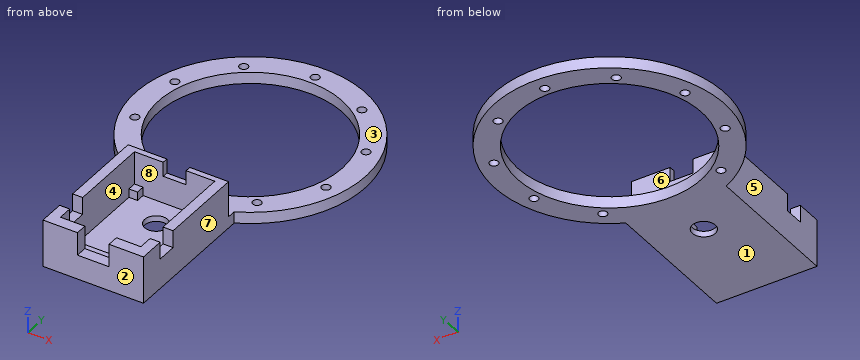
```python
from build123d import *

# Parameters (mm, degrees)
SKETCH1_R             = 1.5
SKETCH1_R_2           = 32
BOSS_EXTRUDE1_DEPTH   = 4
SKETCH1_3_R           = 4
BOSS_EXTRUDE2_DEPTH   = 2
SKETCH1_11_W          = 28
SKETCH1_11_H          = 6
BOSS_EXTRUDE4_DEPTH   = 5
SKETCH1_11_W_2        = 3
SKETCH1_11_H_2        = 3
BOSS_EXTRUDE4_2_DEPTH = 5
BOSS_EXTRUDE4_3_DEPTH = 5
SKETCH1_21_W          = 35
SKETCH1_21_H          = 46
BOSS_EXTRUDE7_DEPTH   = 16.5
SKETCH3_W             = 6
SKETCH3_H             = 7
CUT_EXTRUDE1_DEPTH    = 35.5
SKETCH4_W             = 11
SKETCH4_H             = 8
CUT_EXTRUDE2_DEPTH    = 4
SKETCH5_W             = 8
SKETCH5_H             = 5
CUT_EXTRUDE3_DEPTH    = 52


with BuildPart() as part:
    # Sketch1 → Boss-Extrude1 (new body)
    with BuildSketch(Plane.XY):
        with BuildLine():
            Line((-17.5, -38.96998799), (17.5, -38.96998799))
            Line((17.5, -38.96998799), (17.5, -35.968736425))
            ThreePointArc((17.5, -35.968736425), (0, 40), (-17.5, -35.968736425))
            Line((-17.5, -35.968736425), (-17.5, -38.96998799))
        make_face()
        with Locations((-20.57248383, -28.315594803)):
            Circle(SKETCH1_R, mode=Mode.SUBTRACT)
        with Locations((20.57248383, -28.315594803)):
            Circle(SKETCH1_R, mode=Mode.SUBTRACT)
        with Locations((-33.28697807, -10.815594803)):
            Circle(SKETCH1_R, mode=Mode.SUBTRACT)
        Circle(SKETCH1_R_2, mode=Mode.SUBTRACT)
        with Locations((-33.28697807, 10.815594803)):
            Circle(SKETCH1_R, mode=Mode.SUBTRACT)
        with Locations((-20.57248383, 28.315594803)):
            Circle(SKETCH1_R, mode=Mode.SUBTRACT)
        with Locations((0, 35)):
            Circle(SKETCH1_R, mode=Mode.SUBTRACT)
        with Locations((33.28697807, -10.815594803)):
            Circle(SKETCH1_R, mode=Mode.SUBTRACT)
        with Locations((33.28697807, 10.815594803)):
            Circle(SKETCH1_R, mode=Mode.SUBTRACT)
        with Locations((20.57248383, 28.315594803)):
            Circle(SKETCH1_R, mode=Mode.SUBTRACT)
    extrude(amount=BOSS_EXTRUDE1_DEPTH)



with BuildPart() as body_2:
    # Sketch1<3> → Boss-Extrude2 (new body)
    with BuildSketch(Plane.XY):
        Polygon((11, -40.96998799), (-11, -40.96998799), (-11, -43.96998799), (-14, -43.96998799), (-14, -74.96998799), (14, -74.96998799), (14, -43.96998799), (11, -43.96998799), align=None)
        with Locations((0, -50.96998799)):
            Circle(SKETCH1_3_R, mode=Mode.SUBTRACT)
    extrude(amount=BOSS_EXTRUDE2_DEPTH)


with BuildPart() as body_3:
    # Sketch1<11> → Boss-Extrude4 (new body)
    with BuildSketch(Plane.XY):
        with Locations((0, -77.96998799)):
            Rectangle(SKETCH1_11_W, SKETCH1_11_H)
    extrude(amount=BOSS_EXTRUDE4_DEPTH)


with BuildPart() as body_4:
    # Sketch1<11> → Boss-Extrude4 2 (new body)
    with BuildSketch(Plane.XY):
        with Locations((-12.5, -42.46998799)):
            Rectangle(SKETCH1_11_W_2, SKETCH1_11_H_2)
    extrude(amount=BOSS_EXTRUDE4_2_DEPTH)


with BuildPart() as body_5:
    # Sketch1<11> → Boss-Extrude4 3 (new body)
    with BuildSketch(Plane.XY):
        with Locations((12.5, -42.46998799)):
            Rectangle(SKETCH1_11_W_2, SKETCH1_11_H_2)
    extrude(amount=BOSS_EXTRUDE4_3_DEPTH)


with BuildPart() as part_1:
    add(part.part)

    add(body_2.part)  # Boss-Extrude7 merges body 2

    add(body_3.part)  # Boss-Extrude7 merges body 3

    add(body_4.part)  # Boss-Extrude7 merges body 4

    add(body_5.part)  # Boss-Extrude7 merges body 5
    # Sketch1<21> → Boss-Extrude7 (add)
    with BuildSketch(Plane.XY):
        with Locations((0, -61.96998799)):
            Rectangle(SKETCH1_21_W, SKETCH1_21_H)
        Polygon((-14, -43.96998799), (-14, -40.96998799), (-11, -40.96998799), (11, -40.96998799), (14, -40.96998799), (14, -43.96998799), (14, -74.96998799), (14, -80.96998799), (-14, -80.96998799), (-14, -74.96998799), align=None, mode=Mode.SUBTRACT)
    extrude(amount=BOSS_EXTRUDE7_DEPTH)

    # Sketch3 → Cut-Extrude1 (cut)
    with BuildSketch(Plane(origin=(17.5, 0, 0), x_dir=(0, 0, -1), z_dir=(1, 0, 0))):
        with Locations((-13.5, -72.46998799)):
            Rectangle(SKETCH3_W, SKETCH3_H)
    extrude(amount=-CUT_EXTRUDE1_DEPTH, mode=Mode.SUBTRACT)

    # Sketch4 → Cut-Extrude2 (cut)
    with BuildSketch(Plane(origin=(0, -84.96998799, 0), x_dir=(-1, 0, 0), z_dir=(0, -1, 0))):
        with Locations((0, -12.5)):
            Rectangle(SKETCH4_W, SKETCH4_H)
    extrude(amount=-CUT_EXTRUDE2_DEPTH, mode=Mode.SUBTRACT)

    # Sketch5 → Cut-Extrude3 (cut)
    with BuildSketch(Plane(origin=(0, -84.96998799, 0), x_dir=(-1, 0, 0), z_dir=(0, -1, 0))):
        with Locations((0, -14)):
            Rectangle(SKETCH5_W, SKETCH5_H)
    extrude(amount=-CUT_EXTRUDE3_DEPTH, mode=Mode.SUBTRACT)


solid = part_1.part
```
For this review, take the finished solid that the model builds, in its own axes (mm). Face numbers are marked on the shaded views. A direction names the side the tool comes from. Give positions to 0.01 mm unless a question says otherwise; leave off trailing zeros. Write each loop counter-clockwise with the first axis right and the second up, starting at its lowest first coordinate (ties: lowest second). Pieces come first, ordered by that corner, then holes. Notation, with made-up numbers: M -18.75,79.5 L 29.25,79.5 A24 ccw 29.25,94.5 Z; hole C -8.5,-16.5 d6. An arc over 180 degrees is marked long. Answer as a JSON object with one key per item and string values. Group by question number.
Item 1: For pin 1 Ø0.6 at (y, z) = (-39.5, 14) entering from -X; pin 2 Ø1 at (x, y) = (15, -72.5) entering from +Z; pin 3 Ø2.5 at (x, z) = (-2.5, 3) entering from +Y; pin 4 Ø2.5 at (x, y) = (20.57, 28.32) entering from -Z, all flat-tipped, find the tip position at first contact; note any pin that passes through.
Item 2: Consider section D-D on x = 26. Write out the cut boundary in (y, z).
Item 3: Tool access review of the marked faces 1, 2, 3, 4 and 5: name each direction out of +Z, -Z, +X, -X, +Y, -Y from which nothing blocks a thin tool from reaching the whole face with its end or side.
Item 4: Draft analysis for pull direction Y (two halves, no side actions). For the marked faces 6, 7 and 8, state which applies: +Y half, -Y half, draft (parallel to the pull), parting line (faces both ways), or undercut.
Item 5: Consider section B-B on x = 0. Write out the cut boundary in (y, z), plus the area to 3 significant figures.
Item 6: For probe 1 along Y at (x, z) = (0, 1.2); probe 2 along Y at (x, z) = (6.5, 12.5); probe 3 along X at (y, z) = (-61.5, 13.5), list the stretches that pass through material, from the lowest coordinate up. Write a range as [from, to].
Item 7: Consider section C-C on y = -65. Write out the cut boundary in (x, z).
Item 8: Consider section A-A on z = 13.5. Write out the cut boundary in (x, y).
Check result:
{
 "1": {"pin 1": "stops at x = -17.5", "pin 2": "stops at z = 10.5", "pin 3": "stops at y = 39.98", "pin 4": "passes through"},
 "2": {"outline": "M -30.4,0 L -18.65,0 L -18.65,4 L -30.4,4 Z; M 18.65,0 L 30.4,0 L 30.4,4 L 18.65,4 Z"},
 "3": {"face 1": "-Z, +X, -X, +Y, -Y", "face 2": "+Z, -Z, +X, -X, -Y", "face 3": "+Z, +X, -X, +Y", "face 4": "+Z", "face 5": "+Z, -Z, -X, -Y"},
 "4": {"face 6": "+Y half", "face 7": "draft", "face 8": "undercut"},
 "5": {"outline": "M -84.97,0 L -54.97,0 L -54.97,2 L -74.97,2 L -74.97,5 L -80.97,5 L -80.97,8.5 L -84.97,8.5 Z; M -46.97,0 L -32,0 L -32,4 L -38.97,4 L -38.97,11.5 L -40.97,11.5 L -40.97,2 L -46.97,2 Z; M 32,0 L 33.5,0 L 33.5,4 L 32,4 Z; M 36.5,0 L 40,0 L 40,4 L 36.5,4 Z", "area": "187 mm^2"},
 "6": {"probe 1": "y = [-84.97, -54.97], [-46.97, -32], [32, 33.5], [36.5, 40]", "probe 2": "y = [-84.97, -80.97], [-40.97, -38.97]", "probe 3": "x = [-17.5, -14], [14, 17.5]"},
 "7": {"outline": "M -17.5,0 L 17.5,0 L 17.5,16.5 L 14,16.5 L 14,2 L -14,2 L -14,16.5 L -17.5,16.5 Z"},
 "8": {"outline": "M -17.5,-84.97 L -5.5,-84.97 L -5.5,-80.97 L -14,-80.97 L -14,-75.97 L -17.5,-75.97 Z; M -17.5,-68.97 L -14,-68.97 L -14,-40.97 L -4,-40.97 L -4,-38.97 L -17.5,-38.97 Z; M 4,-40.97 L 14,-40.97 L 14,-68.97 L 17.5,-68.97 L 17.5,-38.97 L 4,-38.97 Z; M 5.5,-84.97 L 17.5,-84.97 L 17.5,-75.97 L 14,-75.97 L 14,-80.97 L 5.5,-80.97 Z"}
}
